The listing builds one solid part. Answer for the finished solid, in the listing's coordinates (mm). A direction names the side the tool comes from. Give positions to 0.01 mm unless a question says otherwise; leave off trailing zeros. Loops run counter-clockwise (first coordinate to the right, second up) from the corner with the lowest first, then second, coordinate; pieces in that order, holes last. Notation, with made-up numbers: (0, 19.5) - (31, 19.5) arc R4 cw to (31, 24.5) - close; hole circle Ø10 at (25, 29). An arc over 180 degrees is marked (long way). Write each question's results on one line, items separated by ' | '.
Autodesk Inventor part; units mm, degrees
ref_plane "YZ Plane" through (0, 0, 0) normal (1, 0, 0) x (0, 1, 0)
ref_plane "XZ Plane" through (0, 0, 0) normal (0, 1, 0) x (-1, 0, 0)
ref_plane "XY Plane" through (0, 0, 0) normal (0, 0, 1) x (1, 0, 0)
sketch "Esquisse3" plane through (0, 0, 0) normal (1, 0, 0) x (0, 1, 0)
  line L0 (0, 0) -> (0, -34.8052)
  line L1 (0, -45) -> (8, -45)
  line L2 (8, -45) -> (8, 0)
  line L3 (0, -45) -> (0, -46.5)
  line L4 (0, -46.5) -> (9.5, -46.5)
  line L5 (8, 0) -> (9.5, 0)
  line L6 (9.5, 0) -> (9.5, -12)
  line L7 (10, -12) -> (10, -17)
  line L8 (9.5, -19) -> (9.5, -46.5)
  line L9 (10, -17) -> (10.5, -17)
  line L10 (10.5, -17) -> (10.5, -17.5)
  line L11 (10.5, -17.5) -> (9.5, -19)
  line L12 (10, -12) -> (9.5, -12)
  dimension "d6" = 1.5
  dimension "d7" = 16
  dimension "d8" = 1.5
  dimension "d10" = 45
  dimension "d16" = 2
  dimension "d17" = 1.5
  dimension "d32" = 0.5
  dimension "d33" = 1.5
  dimension "d34" = 5
  dimension "d35" = 0.5
  dimension "d36" = 12
revolve "Révolution1" add sketch "Esquisse3" angle 360 about axis through (0, 0, 0) along (0, 0, -1)
thread "Filetage2"
chamfer "Chanfrein4" distance 0.5 angle 45 3 edges at (0, -10, -12) (0, -9.5, -46.5) (0, -8, -45)
thread "Filetage3"
equation "\"d6\" = d5"
equation "\"d35\" = d32"
properties part number "cartridge_locker_piston_cyl"
Item 1: A cutting plane is placed at D-D, the plane z = -15. Determine the outline of the cut face in (x, y).
Values found:
outline: circle Ø20 at (0, 0); hole circle Ø16 at (0, 0)
Item 2: A cutting plane is placed at C-C, the plane z = -39. Determine the outline of the cut face in (x, y), plus the area to 3 significant figures.
Values found:
outline: circle Ø19 at (0, 0); hole circle Ø16 at (0, 0) | area: 82.5 mm²
Item 3: For a pull along X with two mould halves and no side action, classify faces 4 (the face through (0, 0, -45)), 5 (the face through (-9, 5, -17)), 6 (the face through (3.2, 10, -17.3)) as released by +X, released by -X, zero draft, split by the parting line, or undercut.
Values found:
face 4: undercut | face 5: zero draft | face 6: split by the parting line
Item 4: Find the intervals of material crossed by line 1 along X through (y, z) = (0, -22.5); line 2 along X through (y, z) = (0, -13); line 3 along Z through (x, y) = (-6.75, 2.75), in increasing order. Write a range as [from, to].
Values found:
line 1: x = [-9.5, -8], [8, 9.5] | line 2: x = [-10, -8], [8, 10] | line 3: z = [-46.5, -45]
Item 5: For faces 1 (the face through (-8.43, 4.38, -32.69)), 2 (the face through (-9.76, -2.17, -14.78)), 3 (the face through (0, 0, -46.5)), determine the directions among +Z, -Z, +X, -X, +Y, -Y from which every point of the face is accessible in a straight line to the end or side of a thin tool.
Values found:
face 1: -Z | face 2: +Z | face 3: -Z, +X, -X, +Y, -Y
Item 6: Flat-ended cylindrical pins translate along their axes: P1, Ø4, axis at x = -5, z = -39.5, coming from the +Y side; P2, Ø5, axis at x = 3, y = 7, coming from the +Z side; P3, Ø12, axis at x = 1, z = -37.5, coming from the -Y side; P4, Ø10, axis at x = 7.5, z = -17, coming from the -Y side. Find the tip coordinate at first contact, or state that the pin passes through.
Values found:
P1: stops at y = 9.01 | P2: stops at z = 0 | P3: stops at y = -9.5 | P4: stops at y = -10.2
